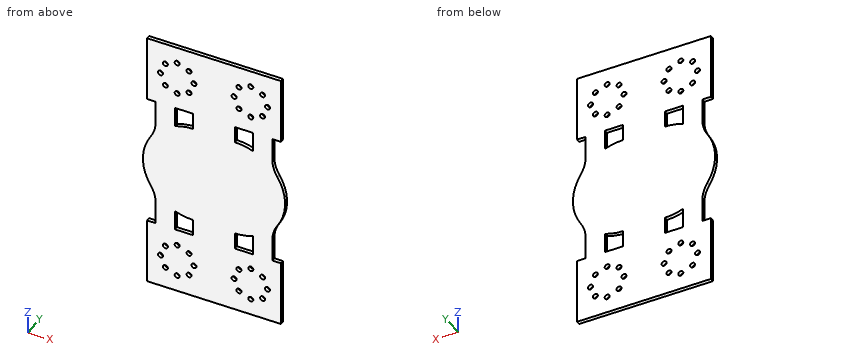
from build123d import *

# Parameters (mm, degrees)
SALIENTE_EXTRUIR1_DEPTH = 2.25
CROQUIS2_R              = 1.5
CORTAR_EXTRUIR1_DEPTH   = 128.323652555
REDONDEO1_R             = 20


with BuildPart() as part:
    # Croquis1 → Saliente-Extruir1 (new body)
    with BuildSketch(Plane(origin=(0, 0, 0), x_dir=(1, 0, 0), z_dir=(0, 1, 0))):
        with BuildLine():
            ThreePointArc((23.270329614, 12), (29.541594579, 15.310243942), (34.860679775, 20))
            ThreePointArc((34.860679775, 20), (42.5, 40), (34.860679775, 60))
            ThreePointArc((34.860679775, 60), (29.541594579, 64.689756058), (23.270329614, 68))
            ThreePointArc((23.270329614, 68), (17.977225575, 69.495762408), (12.5, 70))
            Line((12.5, 70), (12.5, 10))
            ThreePointArc((12.5, 10), (17.977225575, 10.504237592), (23.270329614, 12))
        make_face()
        Polygon((-40, 0), (-40, -40), (40, -40), (40, 0), (34.860679775, 0), (23.270329614, 0), (12.5, 0), (12.5, 10), (12.5, 70), (12.5, 80), (23.270329614, 80), (34.860679775, 80), (40, 80), (40, 120), (-40, 120), (-40, 80), (-34.860679775, 80), (-23.270329614, 80), (-12.5, 80), (-12.5, 70), (-12.5, 40), (-12.5, 10), (-12.5, 0), (-23.270329614, 0), (-34.860679775, 0), align=None)
        with BuildLine():
            ThreePointArc((-34.860679775, 60), (-42.5, 40), (-34.860679775, 20))
            ThreePointArc((-34.860679775, 20), (-29.541594579, 15.310243942), (-23.270329614, 12))
            ThreePointArc((-23.270329614, 12), (-17.977225575, 10.504237592), (-12.5, 10))
            Line((-12.5, 10), (-12.5, 40))
            Line((-12.5, 40), (-12.5, 70))
            ThreePointArc((-12.5, 70), (-17.977225575, 69.495762408), (-23.270329614, 68))
            ThreePointArc((-23.270329614, 68), (-29.541594579, 64.689756058), (-34.860679775, 60))
        make_face()
        with BuildLine():
            Line((23.270329614, 0), (34.860679775, 0))
            Line((34.860679775, 0), (34.860679775, 20))
            ThreePointArc((34.860679775, 20), (29.541594579, 15.310243942), (23.270329614, 12))
            Line((23.270329614, 12), (23.270329614, 0))
        make_face()
        with BuildLine():
            ThreePointArc((23.270329614, 68), (29.541594579, 64.689756058), (34.860679775, 60))
            Line((34.860679775, 60), (34.860679775, 80))
            Line((34.860679775, 80), (23.270329614, 80))
            Line((23.270329614, 80), (23.270329614, 68))
        make_face()
        with BuildLine():
            Line((-34.860679775, 80), (-34.860679775, 60))
            ThreePointArc((-34.860679775, 60), (-29.541594579, 64.689756058), (-23.270329614, 68))
            Line((-23.270329614, 68), (-23.270329614, 80))
            Line((-23.270329614, 80), (-34.860679775, 80))
        make_face()
        with BuildLine():
            Line((-34.860679775, 20), (-34.860679775, 0))
            Line((-34.860679775, 0), (-23.270329614, 0))
            Line((-23.270329614, 0), (-23.270329614, 12))
            ThreePointArc((-23.270329614, 12), (-29.541594579, 15.310243942), (-34.860679775, 20))
        make_face()
    extrude(amount=SALIENTE_EXTRUIR1_DEPTH)

    # Croquis2 → Cortar-Extruir1 (cut, through all)
    with BuildSketch(Plane(origin=(0, 2.25, 0), x_dir=(1, 0, 0), z_dir=(0, 1, 0))):
        with Locations(Location((32, -20, 0), (0, 0, 270))):
            Circle(CROQUIS2_R)
        with Locations(Location((29.071067812, -27.071067812, 0), (0, 0, 270))):
            Circle(CROQUIS2_R)
        with Locations(Location((22, -30, 0), (0, 0, 270))):
            Circle(CROQUIS2_R)
        with Locations(Location((14.928932188, -27.071067812, 0), (0, 0, 270))):
            Circle(CROQUIS2_R)
        with Locations(Location((12, -20, 0), (0, 0, 270))):
            Circle(CROQUIS2_R)
        with Locations(Location((14.928932188, -12.928932188, 0), (0, 0, 270))):
            Circle(CROQUIS2_R)
        with Locations(Location((22, -10, 0), (0, 0, 270))):
            Circle(CROQUIS2_R)
        with Locations(Location((29.071067812, -12.928932188, 0), (0, 0, 270))):
            Circle(CROQUIS2_R)
        with Locations(Location((-29.071067812, -12.928932188, 0), (0, 0, 90))):
            Circle(CROQUIS2_R)
        with Locations(Location((-22, -10, 0), (0, 0, 90))):
            Circle(CROQUIS2_R)
        with Locations(Location((-14.928932188, -12.928932188, 0), (0, 0, 90))):
            Circle(CROQUIS2_R)
        with Locations(Location((-12, -20, 0), (0, 0, 90))):
            Circle(CROQUIS2_R)
        with Locations(Location((-14.928932188, -27.071067812, 0), (0, 0, 90))):
            Circle(CROQUIS2_R)
        with Locations(Location((-22, -30, 0), (0, 0, 90))):
            Circle(CROQUIS2_R)
        with Locations(Location((-29.071067812, -27.071067812, 0), (0, 0, 90))):
            Circle(CROQUIS2_R)
        with Locations(Location((-32, -20, 0), (0, 0, 90))):
            Circle(CROQUIS2_R)
        with Locations(Location((-32, 100, 0), (0, 0, 270))):
            Circle(CROQUIS2_R)
        with Locations(Location((-29.071067812, 107.071067812, 0), (0, 0, 270))):
            Circle(CROQUIS2_R)
        with Locations(Location((-22, 110, 0), (0, 0, 270))):
            Circle(CROQUIS2_R)
        with Locations(Location((-14.928932188, 107.071067812, 0), (0, 0, 270))):
            Circle(CROQUIS2_R)
        with Locations(Location((-12, 100, 0), (0, 0, 270))):
            Circle(CROQUIS2_R)
        with Locations(Location((-14.928932188, 92.928932188, 0), (0, 0, 270))):
            Circle(CROQUIS2_R)
        with Locations(Location((-22, 90, 0), (0, 0, 270))):
            Circle(CROQUIS2_R)
        with Locations(Location((-29.071067812, 92.928932188, 0), (0, 0, 270))):
            Circle(CROQUIS2_R)
        with Locations(Location((29.071067812, 92.928932188, 0), (0, 0, 90))):
            Circle(CROQUIS2_R)
        with Locations(Location((22, 90, 0), (0, 0, 90))):
            Circle(CROQUIS2_R)
        with Locations(Location((14.928932188, 92.928932188, 0), (0, 0, 90))):
            Circle(CROQUIS2_R)
        with Locations(Location((12, 100, 0), (0, 0, 90))):
            Circle(CROQUIS2_R)
        with Locations(Location((14.928932188, 107.071067812, 0), (0, 0, 90))):
            Circle(CROQUIS2_R)
        with Locations(Location((22, 110, 0), (0, 0, 90))):
            Circle(CROQUIS2_R)
        with Locations(Location((29.071067812, 107.071067812, 0), (0, 0, 90))):
            Circle(CROQUIS2_R)
        with Locations(Location((32, 100, 0), (0, 0, 90))):
            Circle(CROQUIS2_R)
    extrude(amount=-CORTAR_EXTRUIR1_DEPTH, mode=Mode.SUBTRACT)

    # Redondeo1
    redondeo1_edges = [part.edges().sort_by_distance(p)[0] for p in [
        (34.860679775, 1.125, -60),
        (34.860679775, 1.125, -20),
        (-34.860679775, 1.125, -20),
        (-34.860679775, 1.125, -60),
    ]]
    fillet(redondeo1_edges, radius=REDONDEO1_R)


solid = part.part
CAD build for the part. Positions are in the model's coordinates, mm. Give positions to 0.01 mm unless a question says otherwise; leave off trailing zeros. Write each loop counter-clockwise with the first axis right and the second up, starting at its lowest first coordinate (ties: lowest second). Pieces come first, ordered by that corner, then holes. Notation, with made-up numbers: M 53,78 L 62,78 A23 cw 62,111 Z; hole C 12,26 d6. An arc over 180 degrees is marked long. Put each result on its own line as item: value. Start each with the question number.
(1) Flat gauge pins, fed straight in: pin 1 Ø1.8 at (x, z) = (12, -100) entering from -Y; pin 2 Ø0.7 at (y, z) = (1, -6.5) entering from +X. Where does each tip first touch, or does it go through?
(2) Band-saw the part on C-C, the plane z = -61.5. Write the cut outline in (x, y).
(3) Band-saw the part on A-A, the plane z = -100. Write the cut outline in (x, y), and give its area (3 significant figures).
(4) Band-saw the part on B-B, the plane y = 1.8. Give the number of separate pieces and of enclosed holes in the cut face, and give its area (3 significant figures).
(5) Probe L1, parallel to X at y = 1.1, z = -90; L2, parallel to Z at x = 29, y = 0.7; L3, parallel to X at y = 1.8, z = -100. List the from-to ranges inside material, lowest first.
Response values:
1. pin 1: passes through
1. pin 2: stops at x = 34.86
2. outline: M -35.51,0 L 35.51,0 L 35.51,2.25 L -35.51,2.25 Z
3. outline: M -40,0 L -33.5,0 L -33.5,2.25 L -40,2.25 Z; M -30.5,0 L -13.5,0 L -13.5,2.25 L -30.5,2.25 Z; M -10.5,0 L 10.5,0 L 10.5,2.25 L -10.5,2.25 Z; M 13.5,0 L 30.5,0 L 30.5,2.25 L 13.5,2.25 Z; M 33.5,0 L 40,0 L 40,2.25 L 33.5,2.25 Z
3. area: 153 mm2
4. separate pieces: 1
4. enclosed holes: 36
4. area: 11,700 mm2
5. L1: x = -40 to -23.5, -20.5 to 20.5, 23.5 to 40
5. L2: z = -120 to -108.57, -105.57 to -94.43, -91.43 to 11.43, 14.43 to 25.57, 28.57 to 40
5. L3: x = -40 to -33.5, -30.5 to -13.5, -10.5 to 10.5, 13.5 to 30.5, 33.5 to 40
